```python
from build123d import *

# Parameters (mm, degrees)
BOSS_EXTRUDE1_DEPTH = 16
FILLET2_R           = 1
SKETCH2_W           = 166
SKETCH2_H           = 295
CUT_EXTRUDE1_DEPTH  = 1
SKETCH3_R           = 2.5
CUT_EXTRUDE2_DEPTH  = 10


with BuildPart() as part:
    # Sketch1 → Boss-Extrude1 (new body)
    with BuildSketch(Plane.XY):
        with BuildLine():
            Line((-94, 165), (94, 165))
            ThreePointArc((94, 165), (101.071067812, 162.071067812), (104, 155))
            Line((104, 155), (104, -155))
            ThreePointArc((104, -155), (101.071067812, -162.071067812), (94, -165))
            Line((94, -165), (-94, -165))
            ThreePointArc((-94, -165), (-101.071067812, -162.071067812), (-104, -155))
            Line((-104, -155), (-104, 155))
            ThreePointArc((-104, 155), (-101.071067812, 162.071067812), (-94, 165))
        make_face()
    extrude(amount=BOSS_EXTRUDE1_DEPTH)

    # Fillet2
    fillet2_edges = [part.edges().sort_by_distance(p)[0] for p in [
        (0, 165, 0),
        (101.071067812, 162.071067812, 0),
        (104, 0, 0),
        (101.071067812, -162.071067812, 0),
        (0, -165, 0),
        (-101.071067812, -162.071067812, 0),
        (-104, 0, 0),
        (-101.071067812, 162.071067812, 0),
    ]]
    fillet(fillet2_edges, radius=FILLET2_R)

    # Sketch2 → Cut-Extrude1 (cut)
    with BuildSketch(Plane.XY.offset(16)):
        Rectangle(SKETCH2_W, SKETCH2_H)
    extrude(amount=-CUT_EXTRUDE1_DEPTH, mode=Mode.SUBTRACT)

    # Sketch3 → Cut-Extrude2 (cut)
    with BuildSketch(Plane(origin=(0, 0, 0), x_dir=(-1, 0, 0), z_dir=(0, 0, -1))):
        with Locations((-50, 50)):
            Circle(SKETCH3_R)
        with Locations((50, 50)):
            Circle(SKETCH3_R)
        with Locations((50, -50)):
            Circle(SKETCH3_R)
        with Locations((-50, -50)):
            Circle(SKETCH3_R)
    extrude(amount=-CUT_EXTRUDE2_DEPTH, mode=Mode.SUBTRACT)


solid = part.part
```
Can you work these out from the model? Positions are in its coordinate system, mm. Coordinates: 2 decimals unless noted, no trailing zeros. Write each loop counter-clockwise with the first axis right and the second up, starting at its lowest first coordinate (ties: lowest second). Pieces come first, ordered by that corner, then holes. Notation, with made-up numbers: M -19,83 L 16,83 A30 cw 16,109 Z; hole C 85.5,47.25 d11. An arc over 180 degrees is marked long. Write item = value, one per line. Start each with the question number.
Q1. I'm going to push flat-ended pins straight in: pin 1 (2.5 mm diameter, centred on x = -51, y = -50.5, fed in from -Z); pin 2 (8 mm diameter, centred on x = 50, y = -50, fed in from +Z); pin 3 (12 mm diameter, centred on x = 32, y = 5.5, fed in from -Z). Where does each tip first touch, or does it pass through?
Q2. If we section it at A-A, the plane y = -95.5: Write out the boundary of the cut face in (x, z), then the cut area to 3 significant figures.
Q3. Thinking about a two-plate mould opening in X: for faces 1 (the face through (-1, 165, 8)), 2 (the face through (104, 2, 8)), 3 (the face through (-1, 2, 15)), which applies, released by +X, released by -X, zero draft, split by the parting line, or undercut?
Q4. If we section it at B-B, the plane x = -56.5: Write out the boundary of the cut face in (y, z), then the cut area to 3 significant figures.
Q5. If I drill on L1, parallel to Y at x = 50, z = 2.25; L2, parallel to Y at x = -71, z = 15.25; L3, parallel to Z at x = 53, y = 4, over which ranges is the centre line in solid material (lowest first)? Write a range as [from, to].
Check sheet entries:
q1.pin_1 = 10
q1.pin_2 = 15
q1.pin_3 = 0
q2.outline = M -104,1 A1 ccw -103,0 L 103,0 A1 ccw 104,1 L 104,16 L 83,16 L 83,15 L -83,15 L -83,16 L -104,16 Z
q2.area = 3,160 mm²
q3.face_1 = zero draft
q3.face_2 = released by +X
q3.face_3 = undercut
q4.outline = M -165,1 A1 ccw -164,0 L 164,0 A1 ccw 165,1 L 165,16 L 147.5,16 L 147.5,15 L -147.5,15 L -147.5,16 L -165,16 Z
q4.area = 4,980 mm²
q5.L1 = [-165, -52.5], [-47.5, 47.5], [52.5, 165]
q5.L2 = [-165, -147.5], [147.5, 165]
q5.L3 = [0, 15]
